The listing builds one solid part. Answer for the finished solid, in the listing's coordinates (mm). A direction names the side the tool comes from. Coordinates: 2 decimals unless noted, no trailing zeros. Loops run counter-clockwise (first coordinate to the right, second up) from the corner with the lowest first, then second, coordinate; pieces in that order, holes last. Notation, with made-up numbers: M 1,74.25 L 15,74.25 A30 cw 15,98.25 Z; hole C -12,87 d11. An arc over 180 degrees is marked long. Return JSON: item names as keys, results as strings. Group by question number.
1. Which of the six approach directions +Z, -Z, +X, -X, +Y, -Y give full straight-line access (tool end or side, diameter ignored) to faces 1 (the face through (-61, 37.6, 1.6)), 2 (the face through (-1, -5, 0)), 3 (the face through (-62.53, -38.364, 1.565)), 4 (the face through (108.43, 40.21, 1.61))?
2. Section C-C (x = 109) is taken. Write down the section's boundary in (y, z) (3 decimals), then the cut area to 3 significant figures.
3. Section D-D (y = -26) is taken. Write down the section's boundary in (x, z) (3 decimals), then the cut area to 3 significant figures.
4. Section A-A (z = 2.1) is taken. Write down the section's boundary in (x, y) (3 decimals).
5. The mould has two halves that part along X. Classify faces 5 (the face through (-1, -5, 3.175)), 6 (the face through (61, -37.6, 1.6)): pulls with the +X half, pulls with the -X half, needs draft (parallel to the pull), parting line crosses it, or undercut.
6. Section B-B (y = 55) is taken. Write down the section's boundary in (x, z) (3 decimals).
7. Straight lines are drawn through the part: L1, parallel to Y at x = -120.65, z = 2.3 (3 decimals); L2, parallel to X at y = 8.5, z = 2.95; L3, parallel to X at y = -28.5, z = 1.7. For each, find the intervals that lie inside material, in ascending order. Write a range as from..to.
8. Given P1, Ø1.5, axis at x = 44, z = 2, coming from the +Y side, flat-ended and moving along its own axis, determine where the tip first touches the part or whether it passes through.
```python
from build123d import *

# Parameters (mm, degrees)
BOSS_EXTRUDE1_DEPTH = 3.175
SKETCH2_R           = 2.286
CUT_EXTRUDE1_DEPTH  = 144.473468802
FILLET1_R           = 12.7


with BuildPart() as part:
    # Sketch1 → Boss-Extrude1 (new body)
    with BuildSketch(Plane.XY):
        with BuildLine():
            Line((-117.810193669, -66.004612663), (0, -7.099515829))
            Line((0, -7.099515829), (117.810193669, -66.004612663))
            ThreePointArc((117.810193669, -66.004612663), (123.988392562, -65.726632633), (127, -60.325))
            Line((127, -60.325), (127, 60.325))
            ThreePointArc((127, 60.325), (123.988392562, 65.726632633), (117.810193669, 66.004612663))
            Line((117.810193669, 66.004612663), (0, 7.099515829))
            Line((0, 7.099515829), (-117.810193669, 66.004612663))
            ThreePointArc((-117.810193669, 66.004612663), (-123.988392562, 65.726632633), (-127, 60.325))
            Line((-127, 60.325), (-127, -60.325))
            ThreePointArc((-127, -60.325), (-123.988392562, -65.726632633), (-117.810193669, -66.004612663))
        make_face()
        Polygon((-114.3, -50.050484171), (-14.199031657, 0), (-114.3, 50.050484171), align=None, mode=Mode.SUBTRACT)
        Polygon((14.199031657, 0), (114.3, 50.050484171), (114.3, -50.050484171), align=None, mode=Mode.SUBTRACT)
    extrude(amount=BOSS_EXTRUDE1_DEPTH)

    # Sketch2 → Cut-Extrude1 (cut, through all)
    with BuildSketch(Plane.XY.offset(3.175)):
        with Locations((-120.65, 60.325)):
            Circle(SKETCH2_R)
        with Locations((-120.65, -60.325)):
            Circle(SKETCH2_R)
        with Locations((120.65, -60.325)):
            Circle(SKETCH2_R)
        with Locations((120.65, 60.325)):
            Circle(SKETCH2_R)
    extrude(amount=-CUT_EXTRUDE1_DEPTH, mode=Mode.SUBTRACT)

    # Fillet1
    fillet1_edges = [part.edges().sort_by_distance(p)[0] for p in [
        (0, -7.099515829, 1.5875),
        (0, 7.099515829, 1.5875),
        (114.3, -50.050484171, 1.5875),
        (114.3, 50.050484171, 1.5875),
        (14.199031657, 0, 1.5875),
        (-14.199031657, 0, 1.5875),
        (-114.3, 50.050484171, 1.5875),
        (-114.3, -50.050484171, 1.5875),
    ]]
    fillet(fillet1_edges, radius=FILLET1_R)


solid = part.part
```
Worked out:
{
 "1": {"face 1": "+Z, -Z, +Y", "face 2": "-Z, +X, -X, +Y, -Y", "face 3": "+Z, -Z, -Y", "face 4": "+Z, -Z"},
 "2": {"outline": "M -61.6,0 L -39.823,0 L -39.823,3.175 L -61.6,3.175 Z; M 39.823,0 L 61.6,0 L 61.6,3.175 L 39.823,3.175 Z", "area": "138 mm^2"},
 "3": {"outline": "M -127,0 L -114.3,0 L -114.3,3.175 L -127,3.175 Z; M -66.199,0 L -37.801,0 L -37.801,3.175 L -66.199,3.175 Z; M 37.801,0 L 66.199,0 L 66.199,3.175 L 37.801,3.175 Z; M 114.3,0 L 127,0 L 127,3.175 L 114.3,3.175 Z", "area": "261 mm^2"},
 "4": {"outline": "M -127,-60.325 A6.35 ccw -117.81,-66.005 L -5.68,-9.939 A12.7 cw 5.68,-9.939 L 117.81,-66.005 A6.35 ccw 127,-60.325 L 127,60.325 A6.35 ccw 117.81,66.005 L 5.68,9.939 A12.7 cw -5.68,9.939 L -117.81,66.005 A6.35 ccw -127,60.325 Z; hole C -120.65,-60.325 d4.572; hole C -120.65,60.325 d4.572; hole M -114.3,-29.501 A12.7 ccw -95.92,-40.861 L -36.917,-11.359 A12.7 ccw -36.917,11.359 L -95.92,40.861 A12.7 ccw -114.3,29.501 Z; hole M 36.917,-11.359 L 95.92,-40.861 A12.7 ccw 114.3,-29.501 L 114.3,29.501 A12.7 ccw 95.92,40.861 L 36.917,11.359 A12.7 ccw Z; hole C 120.65,-60.325 d4.572; hole C 120.65,60.325 d4.572"},
 "5": {"face 5": "needs draft", "face 6": "undercut"},
 "6": {"outline": "M -127,0 L -95.801,0 L -95.801,3.175 L -127,3.175 Z; M 95.801,0 L 127,0 L 127,3.175 L 95.801,3.175 Z"},
 "7": {"L1": "-66.675..-62.611, -58.039..58.039, 62.611..66.675", "L2": "-127..-114.3, -33.16..33.16, 114.3..127", "L3": "-127..-114.3, -71.2..-42.8, 42.8..71.2, 114.3..127"},
 "8": {"P1": "y = 29.47"}
}
